```python
from build123d import *

# Parameters (mm, degrees)
F1_DEPTH = 80
F2_R     = 16
F3_DEPTH = 120


# Not quite as in the source:
# - the program builds the solid bodies; features that only make, move or delete a surface that nothing else refers to are left out


with BuildPart() as f1:
    # F0 (on Front) → F1 (new body)
    with BuildSketch(Plane.XZ):
        Polygon((60, -45), (60, 45), (-60, 45), (-60, -45), (-40, -45), (-40, 30), (40, 30), (40, -45), align=None)
    extrude(amount=F1_DEPTH)

    # F2 (on face) → F3 (cut)
    with BuildSketch(Plane.YZ.offset(60)):
        with BuildLine():
            ThreePointArc((-40.0000000863, -45), (-68.284271278, -33.2842712169), (-80, -5))
            Line((-80, -5), (-80, -45))
            Line((-80, -45), (-40.0000000863, -45))
        make_face()
        with BuildLine():
            Line((0, -45), (0, -5))
            ThreePointArc((0, -5), (-11.7157287831, -33.284271278), (-40.0000000863, -45))
            Line((-40.0000000863, -45), (0, -45))
        make_face()
        with Locations((-40, -5)):
            Circle(F2_R)
    extrude(amount=-F3_DEPTH, mode=Mode.SUBTRACT)


solid = f1.part
```
For this review, take the finished solid that the model builds, in its own axes (mm). A direction names the side the tool comes from. Coordinates: 2 decimals unless noted, no trailing zeros. Loops run counter-clockwise (first coordinate to the right, second up) from the corner with the lowest first, then second, coordinate; pieces in that order, holes last.
1. Insertion check: P1, Ø3, axis at x = 1.5, y = -13.5, coming from the -Z side. The pin has a flat end and moves straight along its axis. Give the tip position at first contact, or say it passes through.
2. Add section D-D, the plane z = -13. Give the boundary of the cut face in (x, y).
3. Add section B-B, the plane y = -31.5. Give the boundary of the cut face in (x, z).
4. Mouldability with a two-part tool opening along Z and no side actions: class faces 3 (the cylindrical face through (50.14, -55.985, -4.297)), 4 (the flat face through (1, -39, 45)), 5 (the flat face through (-60, -31, 11)) as +Z half, -Z half, draft (parallel to the pull), parting line (faces both ways), or undercut.
5. Add section A-A, the plane z = 26. Give the boundary of the cut face in (x, y), then the cut area to 3 significant figures.
6. For faces 1 (the flat face through (-1, 0, 31)), 2 (the flat face through (-40, -31, 9)), list the 3-axis set-ups (+Z, -Z, +X, -X, +Y, -Y) from which the entire face can be reached by the end or side of a thin tool; tool diameter is ignored.
7. Add section C-C, the plane x = 48.5. Give the boundary of the cut face in (y, z), then the cut area to 3 significant figures.
8. For line 1 (Z direction, x = -54.5, y = -40); line 2 (X direction, y = -38.5, z = 29.5); line 3 (Z direction, x = 3, y = -20.5), list the stretches that pass through material, from the lowest coordinate up.
Result:
1. P1: stops at z = 30
2. outline: (-60, -79.19) - (-40, -79.19) - (-40, -53.86) - (-60, -53.86) - close; (-60, -26.14) - (-40, -26.14) - (-40, -0.81) - (-60, -0.81) - close; (40, -79.19) - (60, -79.19) - (60, -53.86) - (40, -53.86) - close; (40, -26.14) - (60, -26.14) - (60, -0.81) - (40, -0.81) - close
3. outline: (-60, -44.09) - (-40, -44.09) - (-40, -18.56) - (-60, -18.56) - close; (-60, 8.56) - (-40, 8.56) - (-40, 30) - (40, 30) - (40, 8.56) - (60, 8.56) - (60, 45) - (-60, 45) - close; (40, -44.09) - (60, -44.09) - (60, -18.56) - (40, -18.56) - close
4. face 3: undercut
4. face 4: +Z half
4. face 5: draft
5. outline: (-60, -80) - (-40, -80) - (-40, 0) - (-60, 0) - close; (40, -80) - (60, -80) - (60, 0) - (40, 0) - close
5. area: 3,200 mm2
6. face 1: +Z, -Z, +X, -X, +Y
6. face 2: -Z, +Y, -Y
7. outline: (-80, -5) arc R40 ccw to (0, -5) - (0, 45) - (-80, 45) - close; hole circle Ø32 at (-40, -5)
7. area: 5,710 mm2
8. line 1: z = -45 to -21, 11 to 45
8. line 2: x = -60 to -40, 40 to 60
8. line 3: z = 30 to 45
